Design review of the part built by this model. Coordinates are the model's own, in mm. A direction names the side the tool comes from. Round coordinates to 2 decimals unless told otherwise and drop trailing zeros. Loops run counter-clockwise (first coordinate to the right, second up) from the corner with the lowest first, then second, coordinate; pieces in that order, holes last. Notation, with made-up numbers: M -34.75,16 L 22.25,16 A18 ccw 22.25,20 Z; hole C -35.5,14.25 d7. An arc over 180 degrees is marked long. One line per item, written item: value. Start each with the question number.
Item 1: We need section B-B (z = 43.5). Write out the cut boundary in (x, y), then the cut area to 3 significant figures.
Item 2: We need section A-A (x = 35). Write out the cut boundary in (y, z).
Item 3: We need section C-C (y = 21). Write out the cut boundary in (x, z), then the cut area to 3 significant figures.
Item 4: Mouldability with a two-part tool opening along Y and no side actions: class faces 1 (the flat face through (0, 35, 1)), 2 (the flat face through (-50, 25, -1)), 3 (the flat face through (34, 15.7, 1)), 4 (the flat face through (0, 8, -40)) as released by +Y, released by -Y, zero draft, split by the parting line, or undercut.
Item 5: For faces 5 (the flat face through (0, 8, 40)), 6 (the flat face through (1, 25, 60)), 7 (the flat face through (25, 8, -1)), list the 3-axis set-ups (+Z, -Z, +X, -X, +Y, -Y) from which the entire face can be reached by the end or side of a thin tool; tool diameter is ignored.
Item 6: Clearance check with flat-ended pins moving along their axes: pin 1 (12.5 mm diameter, centred on x = -4, y = 10.5, fed in from +Z); pin 2 (4.5 mm diameter, centred on y = 8.5, z = 9.5, fed in from -X); pin 3 (6 mm diameter, centred on x = -13, y = 29.5, fed in from -Z); pin 4 (17.5 mm diameter, centred on y = 8, z = -10, fed in from +X). State where each tip first meets the part, or that it passes through.
Item 7: We need section D-D (x = 61). Write out the cut boundary in (y, z), then the cut area to 3 significant figures.
Item 8: For line 1 along Y through (x, z) = (-41, -2.5); line 2 along Y through (x, z) = (-78, -103.5); line 3 along X through (y, z) = (14, 39), list the stretches that pass through material, from the lowest coordinate up.
from build123d import *

# Parameters (mm, degrees)
F0_W     = 195
F0_H     = 318
F1_DEPTH = 95
F2_W     = 50
F2_H     = 80
F3_DEPTH = 35
F4_START = 15.7
F2_W_2   = 100
F2_H_2   = 120
F4_DEPTH = 19.2


with BuildPart() as f1:
    # F0 (on Front) → F1 (new body)
    with BuildSketch(Plane.XZ):
        Rectangle(F0_W, F0_H)
    extrude(amount=F1_DEPTH)

    # F2 (on face) → F3 (join)
    with BuildSketch(Plane(origin=(0, 0, 0), x_dir=(-1, 0, 0), z_dir=(0, 1, 0))):
        Rectangle(F2_W, F2_H)
    extrude(amount=F3_DEPTH)

    # F2 (on face) → F4 (join)
    with BuildSketch(Plane(origin=(0, 0, 0), x_dir=(-1, 0, 0), z_dir=(0, 1, 0)).offset(F4_START)):
        Rectangle(F2_W_2, F2_H_2)
        Rectangle(F2_W, F2_H, mode=Mode.SUBTRACT)
    extrude(amount=F4_DEPTH)


solid = f1.part
A:
1. outline: M -97.5,-95 L 97.5,-95 L 97.5,0 L -97.5,0 Z; M -50,15.7 L 50,15.7 L 50,34.9 L -50,34.9 Z
1. area: 20,400 mm2
2. outline: M -95,-159 L 0,-159 L 0,159 L -95,159 Z; M 15.7,-60 L 34.9,-60 L 34.9,60 L 15.7,60 Z
3. outline: M -50,-60 L 50,-60 L 50,60 L -50,60 Z
3. area: 12,000 mm2
4. face 1: released by +Y
4. face 2: zero draft
4. face 3: undercut
4. face 4: undercut
5. face 5: +Z, +X, -X
5. face 6: +Z, +X, -X, +Y
5. face 7: +Z, -Z, +X
6. pin 1: z = 60
6. pin 2: x = -25
6. pin 3: z = -60
6. pin 4: x = 97.5
7. outline: M -95,-159 L 0,-159 L 0,159 L -95,159 Z
7. area: 30,200 mm2
8. line 1: -95 to 0, 15.7 to 34.9
8. line 2: -95 to 0
8. line 3: -25 to 25
